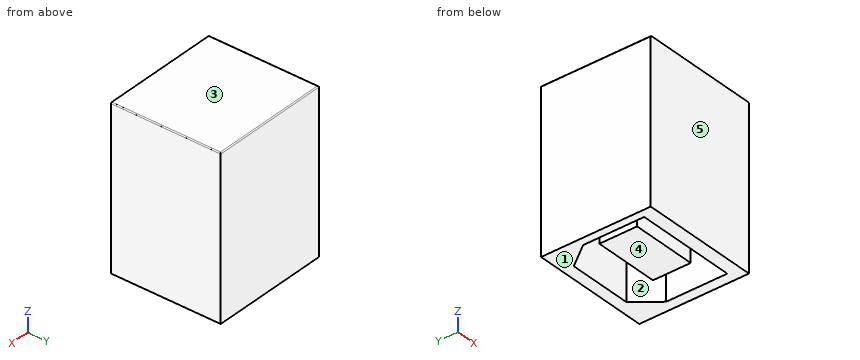
```python
from build123d import *

# Parameters (mm, degrees)
SKETCH1_W           = 12
SKETCH1_H           = 16
BOSS_EXTRUDE1_DEPTH = 11
CUT_EXTRUDE1_DEPTH  = 11
FILLET1_R           = 0.1
SKETCH5_W           = 6.545638519
SKETCH5_H           = 3.78409842
BOSS_EXTRUDE2_DEPTH = 10


with BuildPart() as part:
    # Sketch1 → Boss-Extrude1 (new body)
    with BuildSketch(Plane(origin=(0, 0, 0), x_dir=(1, 0, 0), z_dir=(0, 1, 0))):
        Rectangle(SKETCH1_W, SKETCH1_H)
    extrude(amount=BOSS_EXTRUDE1_DEPTH)

    # Sketch4 → Cut-Extrude1 (cut)
    with BuildSketch(Plane(origin=(0, 0, -8), x_dir=(-1, 0, 0), z_dir=(0, 0, -1))):
        Polygon((-4.942176734, 1.304641084), (5.205759493, 1.304641084), (5.205759493, 7.432940234), (3.404610639, 9.849115526), (-3.0092365, 9.849115526), (-4.942176734, 7.432940234), align=None)
    extrude(amount=-CUT_EXTRUDE1_DEPTH, mode=Mode.SUBTRACT)

    # Fillet1
    fillet1_edges = [part.edges().sort_by_distance(p)[0] for p in [
        (0, 11, 8),
        (6, 5.5, 8),
        (-6, 5.5, 8),
    ]]
    fillet(fillet1_edges, radius=FILLET1_R)

    # Sketch5 → Boss-Extrude2 (add)
    with BuildSketch(Plane(origin=(0, 0, 3), x_dir=(-1, 0, 0), z_dir=(0, 0, -1))):
        with Locations((0.13179138, 5.389997139)):
            Rectangle(SKETCH5_W, SKETCH5_H)
    extrude(amount=BOSS_EXTRUDE2_DEPTH)


solid = part.part
```
Work out the finished part from the listing and answer in its coordinate system (mm). Face numbers are marked on the shaded views. A direction names the side the tool comes from. Coordinates: 2 decimals unless noted, no trailing zeros. Loops run counter-clockwise (first coordinate to the right, second up) from the corner with the lowest first, then second, coordinate; pieces in that order, holes last. Notation, with made-up numbers: (22, 63.5) - (35, 63.5) arc R24 cw to (35, 83.5) - close; hole circle Ø8 at (37, 12). An arc over 180 degrees is marked (long way). Use a Markdown table: item, result.
Item 1: The mould has two halves that part along Y. Classify the marked faces 3, 4 and 5: +Y half, -Y half, draft (parallel to the pull), parting line (faces both ways), or undercut.
Evaluation:
| item | result |
|---|---|
| face 3 | draft |
| face 4 | undercut |
| face 5 | -Y half |
Item 2: Find section A-A, the plane z = -6.5. Determine the outline of the cut face in (x, y).
Evaluation:
| item | result |
|---|---|
| outline | (-6, 0) - (6, 0) - (6, 11) - (-6, 11) - close; (-3.4, 3.5) - (3.14, 3.5) - (3.14, 7.28) - (-3.4, 7.28) - close; hole (-5.21, 1.3) - (4.94, 1.3) - (4.94, 7.43) - (3.01, 9.85) - (-3.4, 9.85) - (-5.21, 7.43) - close |
Item 3: For the marked faces 1 and 2, determine the directions among +Z, -Z, +X, -X, +Y, -Y from which every point of the face is accessible in a straight line to the end or side of a thin tool.
Evaluation:
| item | result |
|---|---|
| face 1 | -Z, +X, -X, +Y, -Y |
| face 2 | -Z |
Item 4: Given pin 1 Ø3 at (x, z) = (0, -1) entering from -Y; pin 2 Ø1.1 at (x, y) = (-1.5, 4.5) entering from -Z, each flat-ended and moving along its own axis, determine where each tip first touches the part or whether it passes through.
Evaluation:
| item | result |
|---|---|
| pin 1 | stops at y = 0 |
| pin 2 | stops at z = -7 |
Item 5: Consider probe 1 along Y at (x, z) = (1, -0.5); probe 2 along X at (y, z) = (6.75, -1.5); probe 3 along X at (y, z) = (3.25, 2.25). Determine where each line is inside the solid, lowest interval first. Write a range as from..to.
Evaluation:
| item | result |
|---|---|
| probe 1 | y = 0..1.3, 3.5..7.28, 9.85..11 |
| probe 2 | x = -6..-5.21, -3.4..3.14, 4.94..6 |
| probe 3 | x = -6..-5.21, 4.94..6 |
Item 6: Find section D-D, the plane y = 2.5. Determine the outline of the cut face in (x, z).
Evaluation:
| item | result |
|---|---|
| outline | (-6, -8) - (-5.21, -8) - (-5.21, 3) - (4.94, 3) - (4.94, -8) - (6, -8) - (6, 7.9) arc R0.1 ccw to (5.9, 8) - (-5.9, 8) arc R0.1 ccw to (-6, 7.9) - close |
Item 7: Find section C-C, the plane x = 2. Determine the outline of the cut face in (y, z).
Evaluation:
| item | result |
|---|---|
| outline | (0, -8) - (1.3, -8) - (1.3, 3) - (3.5, 3) - (3.5, -7) - (7.28, -7) - (7.28, 3) - (9.85, 3) - (9.85, -8) - (11, -8) - (11, 7.9) arc R0.1 ccw to (10.9, 8) - (0, 8) - close |
Item 8: Find section B-B, the plane y = 4.75. Determine the outline of the cut face in (x, z), and give its area (3 significant figures).
Evaluation:
| item | result |
|---|---|
| outline | (-6, -8) - (-5.21, -8) - (-5.21, 3) - (-3.4, 3) - (-3.4, -7) - (3.14, -7) - (3.14, 3) - (4.94, 3) - (4.94, -8) - (6, -8) - (6, 7.9) arc R0.1 ccw to (5.9, 8) - (-5.9, 8) arc R0.1 ccw to (-6, 7.9) - close |
| area | 146 mm2 |
